from build123d import *

# Parameters (mm, degrees)
SKETCH_1_W          = 15
SKETCH_1_H          = 40
EXTRUDE_1_DEPTH     = 32
SKETCH_3_W          = 15
SKETCH_3_H          = 32
EXTRUDE_2_DEPTH     = 10
SKETCH_5_W          = 13
SKETCH_5_H          = 45
CUT_EXTRUDE_1_DEPTH = 62.229078059
SKETCH_7_W          = 32
SKETCH_7_H          = 50
EXTRUDE_3_DEPTH     = 5
SKETCH_8_W          = 3
SKETCH_8_H          = 40
CUT_EXTRUDE_2_DEPTH = 63.641839053
SKETCH_9_W          = 3
SKETCH_9_H          = 5
CUT_EXTRUDE_3_DEPTH = 63.641839053
SKETCH_10_R         = 1.5
EXTRUDE_4_DEPTH     = 5
SKETCH_11_R         = 1.05
CUT_EXTRUDE_4_DEPTH = 63.641839053
SKETCH_12_W         = 4
SKETCH_12_H         = 5
CUT_EXTRUDE_5_DEPTH = 63.641839053
SKETCH_13_W         = 2.538060983
SKETCH_13_H         = 40
CUT_EXTRUDE_6_DEPTH = 63.641839053
SKETCH_14_W         = 20
SKETCH_14_H         = 2
CUT_EXTRUDE_7_DEPTH = 63.641839053


with BuildPart() as part:
    # 草图1 → 凸台-拉伸1 (new body)
    with BuildSketch(Plane.XY):
        with Locations((7.5, 20)):
            Rectangle(SKETCH_1_W, SKETCH_1_H)
    extrude(amount=EXTRUDE_1_DEPTH)

    # 草图3 → 凸台-拉伸2 (add)
    with BuildSketch(Plane(origin=(0, 40, 0), x_dir=(1, 0, 0), z_dir=(0, 1, 0))):
        with Locations((7.5, -16)):
            Rectangle(SKETCH_3_W, SKETCH_3_H)
    extrude(amount=EXTRUDE_2_DEPTH)

    # 草图5 → 切除-拉伸1 (cut, through all)
    with BuildSketch(Plane.XY.offset(32)):
        with Locations((6.5, 22.5)):
            Rectangle(SKETCH_5_W, SKETCH_5_H)
    extrude(amount=-CUT_EXTRUDE_1_DEPTH, mode=Mode.SUBTRACT)

    # 草图7 → 凸台-拉伸3 (add)
    with BuildSketch(Plane(origin=(15, 0, 0), x_dir=(0, 0, -1), z_dir=(1, 0, 0))):
        with Locations((-16, 25)):
            Rectangle(SKETCH_7_W, SKETCH_7_H)
    extrude(amount=EXTRUDE_3_DEPTH)

    # 草图8 → 切除-拉伸2 (cut, through all)
    with BuildSketch(Plane.XY.offset(32)):
        with Locations((14.5, 25)):
            Rectangle(SKETCH_8_W, SKETCH_8_H)
    extrude(amount=-CUT_EXTRUDE_2_DEPTH, mode=Mode.SUBTRACT)

    # 草图9 → 切除-拉伸3 (cut, through all)
    with BuildSketch(Plane.XY.offset(32)):
        with Locations((14.5, 2.5)):
            Rectangle(SKETCH_9_W, SKETCH_9_H)
    extrude(amount=-CUT_EXTRUDE_3_DEPTH, mode=Mode.SUBTRACT)

    # 草图10 → 凸台-拉伸4 (add)
    with BuildSketch(Plane.XZ.offset(-45)):
        with Locations(Location((3, 16, 0), (0, 0, 90))):
            Circle(SKETCH_10_R)
    extrude(amount=EXTRUDE_4_DEPTH)

    # 草图11 → 切除-拉伸4 (cut, through all)
    with BuildSketch(Plane(origin=(20, 0, 0), x_dir=(0, 0, -1), z_dir=(1, 0, 0))):
        with Locations((-24, 34.2)):
            Circle(SKETCH_11_R)
        with Locations((-24, 26.2)):
            Circle(SKETCH_11_R)
        with Locations((-24, 18.2)):
            Circle(SKETCH_11_R)
        with Locations((-16, 34.2)):
            Circle(SKETCH_11_R)
        with Locations((-16, 26.2)):
            Circle(SKETCH_11_R)
        with Locations((-16, 18.2)):
            Circle(SKETCH_11_R)
        with Locations((-8, 18.2)):
            Circle(SKETCH_11_R)
        with Locations((-8, 26.2)):
            Circle(SKETCH_11_R)
        with Locations((-8, 34.2)):
            Circle(SKETCH_11_R)
    extrude(amount=-CUT_EXTRUDE_4_DEPTH, mode=Mode.SUBTRACT)

    # 草图12 → 切除-拉伸5 (cut, through all)
    with BuildSketch(Plane.XY.offset(32)):
        with Locations((18, 2.5)):
            Rectangle(SKETCH_12_W, SKETCH_12_H)
    extrude(amount=-CUT_EXTRUDE_5_DEPTH, mode=Mode.SUBTRACT)

    # 草图13 → 切除-拉伸6 (cut, through all)
    with BuildSketch(Plane.XY.offset(32)):
        with Locations((17.269030492, 25)):
            Rectangle(SKETCH_13_W, SKETCH_13_H)
    extrude(amount=-CUT_EXTRUDE_6_DEPTH, mode=Mode.SUBTRACT)

    # 草图14 → 切除-拉伸7 (cut, through all)
    with BuildSketch(Plane.XY.offset(32)):
        with Locations((10, 49)):
            Rectangle(SKETCH_14_W, SKETCH_14_H)
    extrude(amount=-CUT_EXTRUDE_7_DEPTH, mode=Mode.SUBTRACT)


solid = part.part
Can you work these out from the model? Positions are in its coordinate system, mm. A direction names the side the tool comes from. Round coordinates to 2 decimals unless told otherwise and drop trailing zeros. Loops run counter-clockwise (first coordinate to the right, second up) from the corner with the lowest first, then second, coordinate; pieces in that order, holes last. Notation, with made-up numbers: (28, 24.5) - (86, 24.5) arc R12 cw to (86, 34.5) - close; hole circle Ø4 at (-12, 64). An arc over 180 degrees is marked (long way). Write item = value, one per line. Start each with the question number.
(1) If we section it at D-D (z = 30.5): Please give me the cut outline in (x, y).
(2) If we section it at B-B (z = 8): Please give me the cut outline in (x, y).
(3) If we section it at A-A (y = 18.2): Please give me the cut outline in (x, z), and give its area (3 significant figures).
(4) If we section it at C-C (z = 16): Please give me the cut outline in (x, y).
(5) If we mould it in two halves opening along Y, with no side actions, what happens to faces 1 (the face through (19, 5, 16)), 2 (the face through (19.28, 27.24, 24.14)), 3 (the face through (19, 36, 0))? For each: released by +Y, released by -Y, zero draft, split by the parting line, or undercut.
(6) If I drill on probe 1 along Y at (x, z) = (19.45, 16); probe 2 along X at (y, z) = (18.5, 13); probe 3 along Y at (x, z) = (15, 23.5), over which ranges is the centre line in solid material (lowest first)? Write a range as [from, to].
(7) For P1, Ø1.5, axis at x = 2.5, z = 16.5, coming from the -Y side; P2, Ø1.3, axis at y = 26.2, z = 8, coming from the +X side; P3, Ø10, axis at y = 18, z = 11, coming from the -X side; P4, Ø5.5, axis at x = 7.5, z = 15.5, coming from the -Y side, each with a flat end and sliding along its axis, tell me the tip position at first contact or that it passes through.
(8) For faces 4 (the face through (2.93, 42.54, 14.5)), 5 (the face through (19.28, 19.24, 16.14)), 6 (the face through (3, 40, 16)), which set-ups out of +Z, -Z, +X, -X, +Y, -Y let a thin tool reach every point of the face, with its end or its side?
Ans:
q1.outline = (0, 45) - (18.54, 45) - (18.54, 5) - (20, 5) - (20, 48) - (0, 48) - close
q2.outline = (0, 45) - (18.54, 45) - (18.54, 35.25) - (20, 35.25) - (20, 48) - (0, 48) - close; (18.54, 5) - (20, 5) - (20, 17.15) - (18.54, 17.15) - close; (18.54, 19.25) - (20, 19.25) - (20, 25.15) - (18.54, 25.15) - close; (18.54, 27.25) - (20, 27.25) - (20, 33.15) - (18.54, 33.15) - close
q3.outline = (18.54, 0) - (20, 0) - (20, 6.95) - (18.54, 6.95) - close; (18.54, 9.05) - (20, 9.05) - (20, 14.95) - (18.54, 14.95) - close; (18.54, 17.05) - (20, 17.05) - (20, 22.95) - (18.54, 22.95) - close; (18.54, 25.05) - (20, 25.05) - (20, 32) - (18.54, 32) - close
q3.area = 37.6 mm²
q4.outline = (0, 45) - (1.5, 45) - (1.5, 40) - (4.5, 40) - (4.5, 45) - (18.54, 45) - (18.54, 35.25) - (20, 35.25) - (20, 48) - (0, 48) - close; (18.54, 5) - (20, 5) - (20, 17.15) - (18.54, 17.15) - close; (18.54, 19.25) - (20, 19.25) - (20, 25.15) - (18.54, 25.15) - close; (18.54, 27.25) - (20, 27.25) - (20, 33.15) - (18.54, 33.15) - close
q5.face_1 = released by -Y
q5.face_2 = undercut
q5.face_3 = zero draft
q6.probe_1 = [5, 17.15], [19.25, 25.15], [27.25, 33.15], [35.25, 48]
q6.probe_2 = [18.54, 20]
q6.probe_3 = [45, 48]
q7.P1 = 40
q7.P2 = through
q7.P3 = 18.54
q7.P4 = 45
q8.face_4 = -Y
q8.face_5 = +X, -X
q8.face_6 = +Z, -Z, -X, -Y
